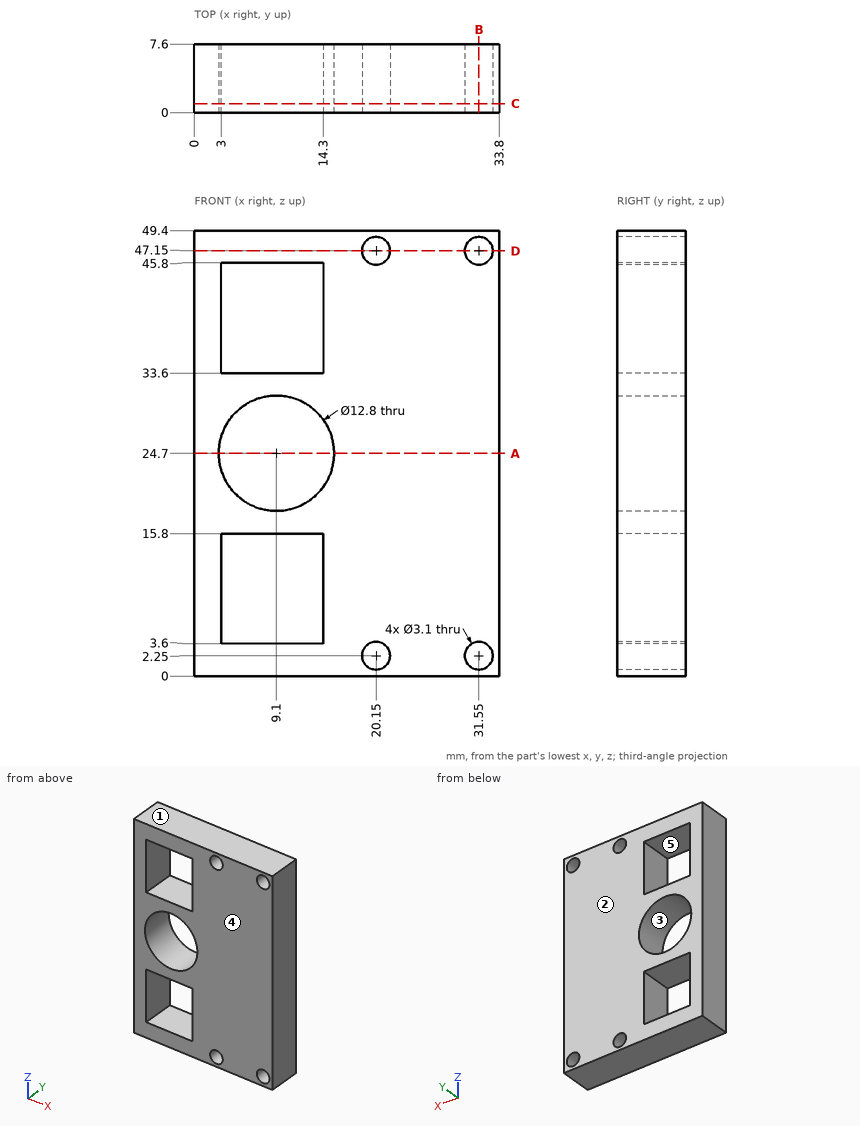
Design review of the part shown in the three views and the two pictorial views. Dimensions are in mm from the part's minimum x, y and z. A direction names the side the tool comes from. Give positions to 0.01 mm unless a question says otherwise; leave off trailing zeros. Order: outer loops, then holes, each group sorted by start corner. A loop starts at its lowest first (then second) coordinate and runs counter-clockwise, first axis right, second up. Notation, with made-up numbers: M 9.5,5.25 L 31.5,5.25 A23 ccw 31.5,34.25 Z; hole C 57.5,18.25 d7. An arc over 180 degrees is marked long. Answer in a Markdown table with one row per item. Add a question column.
(1) Consider section D-D on z = 47.15. State the section outline as (x, y) points, and give its area (3 significant figures).
(2) Mouldability with a two-part tool opening along Z and no side actions: class the marked faces 1, 2 and 3 as +Z half, -Z half, draft (parallel to the pull), parting line (faces both ways), or undercut.
(3) Consider section A-A on z = 24.7. State the section outline as (x, y) points.
(4) Consider section C-C on y = 1. State the section outline as (x, z) points.
(5) For the marked faces 4 and 5, list the 3-axis set-ups (+Z, -Z, +X, -X, +Y, -Y) from which the entire face can be reached by the end or side of a thin tool; tool diameter is ignored.
(6) Wall thickness on probe 1 along X at (y, z) = (5.75, 2.25); probe 2 along Z at (x, y) = (20.15, 2.5); probe 3 along Z at (x, y) = (9.1, 2.5): over which ranges is each line inside the solid? List them lowest first. Write a range as [from, to].
(7) For pin 1 (1.5 mm diameter, centred on x = 18, z = 32, fed in from -Y), flat-tipped, find the tip position at first contact; note if it passes through.
(8) Consider section B-B on x = 31.55. State the section outline as (y, z) points.
Evaluation:
| question | item | result |
|---|---|---|
| 1 | outline | M 0,0 L 18.6,0 L 18.6,7.6 L 0,7.6 Z; M 21.7,0 L 30,0 L 30,7.6 L 21.7,7.6 Z; M 33.1,0 L 33.8,0 L 33.8,7.6 L 33.1,7.6 Z |
| 1 | area | 210 mm^2 |
| 2 | face 1 | +Z half |
| 2 | face 2 | draft |
| 2 | face 3 | undercut |
| 3 | outline | M 0,0 L 2.7,0 L 2.7,7.6 L 0,7.6 Z; M 15.5,0 L 33.8,0 L 33.8,7.6 L 15.5,7.6 Z |
| 4 | outline | M 0,0 L 33.8,0 L 33.8,49.4 L 0,49.4 Z; hole C 9.1,24.7 d12.8; hole M 3,3.6 L 14.3,3.6 L 14.3,15.8 L 3,15.8 Z; hole M 3,33.6 L 14.3,33.6 L 14.3,45.8 L 3,45.8 Z; hole C 20.15,2.25 d3.1; hole C 20.15,47.15 d3.1; hole C 31.55,2.25 d3.1; hole C 31.55,47.15 d3.1 |
| 5 | face 4 | +Z, -Z, +X, -X, -Y |
| 5 | face 5 | +Y, -Y |
| 6 | probe 1 | x = [0, 18.6], [21.7, 30], [33.1, 33.8] |
| 6 | probe 2 | z = [0, 0.7], [3.8, 45.6], [48.7, 49.4] |
| 6 | probe 3 | z = [0, 3.6], [15.8, 18.3], [31.1, 33.6], [45.8, 49.4] |
| 7 | pin 1 | stops at y = 0 |
| 8 | outline | M 0,0 L 7.6,0 L 7.6,0.7 L 0,0.7 Z; M 0,3.8 L 7.6,3.8 L 7.6,45.6 L 0,45.6 Z; M 0,48.7 L 7.6,48.7 L 7.6,49.4 L 0,49.4 Z |
